CAD build for the part. Positions are in the model's coordinates, mm. Face numbers are marked on the shaded views. A direction names the side the tool comes from. Round coordinates to 2 decimals unless told otherwise and drop trailing zeros. Write each loop counter-clockwise with the first axis right and the second up, starting at its lowest first coordinate (ties: lowest second). Pieces come first, ordered by that corner, then holes. Notation, with made-up numbers: (67.25, 20.25) - (93.25, 20.25) arc R14 cw to (93.25, 24.25) - close; hole circle Ø3 at (44.5, 61). An arc over 180 degrees is marked (long way). Put each result on its own line as item: value. Start each with the question number.
Item 1: Drill centre lines: line 1 (X direction, y = 12.35, z = -58); line 2 (Z direction, x = 66.5, y = 4.5); line 3 (Z direction, x = 46.5, y = 2.5). Where is each one in solid material? Low to high. Write a range as from..to.
Item 2: Cut at B-B (z = 3). Give the cut face in (x, y).
Item 3: Cut at C-C (z = -33). Give the cut face in (x, y), and give its area (3 significant figures).
Item 4: Mould opens along Z. For the marked faces 1, 2, 3 and 4 say: released by +Z, released by -Z, zero draft, split by the parting line, or undercut.
Item 5: Cut at A-A (y = 8). Give the cut face in (x, z).
Item 6: Cut at D-D (x = 47.5). Give the cut face in (y, z).
Item 7: 3-axis set-ups, long thin cutter, end or side, ignore diameter. For the marked faces 5, 6 and 7: which of +Z, -Z, +X, -X, +Y, -Y reach the whole face in a straight line?
Item 8: Pin check, flat tips, straight feed: pin 1 Ø5 at (y, z) = (10, -6) entering from -X; pin 2 Ø4 at (x, z) = (16.5, -25.5) entering from +Y; pin 3 Ø8.5 at (x, y) = (52.5, 6) entering from +Z. Stop position of each tip, or through.
```python
from build123d import *

# Parameters (mm, degrees)
BOSS_EXTRUDE1_DEPTH          = 30
SHELL2_T                     = 3
CUT_EXTRUDE2_REACH           = 183.177
BOSS_EXTRUDE5_DEPTH          = 25.5
SKETCH17_W                   = 8
SKETCH17_H                   = 25.58
BOSS_EXTRUDE6_DEPTH          = 5
CUT_EXTRUDE3_REACH           = 182.934
SKETCH18_R                   = 1.75
SKETCH20_W                   = 197.48203017
SKETCH20_H                   = 83.172325934
CUT_EXTRUDE4_DEPTH           = 16.5
CUT_EXTRUDE5_REACH           = 180.984
OUTLINE_OF_MOTOR_PRESS_FIT_W = 41.4
OUTLINE_OF_MOTOR_PRESS_FIT_H = 20.5
SKETCH24_W                   = 46.48
SKETCH24_H                   = 2.54
BOSS_EXTRUDE7_DEPTH          = 1
CUT_EXTRUDE6_DEPTH           = 180.263074837
CUT_EXTRUDE6_DEPTH_BACK      = 180.263074837
SKETCH26_W                   = 55
SKETCH26_H                   = 13.5
BOSS_EXTRUDE8_DEPTH          = 3
FILLET1_R                    = 25
FILLET2_R                    = 25
SKETCH28_W                   = 6
SKETCH28_H                   = 6
SKETCH28_R                   = 1.75
BOSS_EXTRUDE9_DEPTH          = 2.5
FILLET3_R                    = 1
FILLET4_R                    = 10
CUT_EXTRUDE7_REACH           = 95.975
SKETCH30_R                   = 1.3


with BuildPart() as part:
    # Sketch1 → Boss-Extrude1 (new body)
    with BuildSketch(Plane(origin=(0, 0, 0), x_dir=(1, 0, 0), z_dir=(0, 1, 0))):
        Polygon((0, 46), (9, 55), (161, 55), (170, 46), (170, 9), (161, 0), (9, 0), (0, 9), align=None)
    extrude(amount=BOSS_EXTRUDE1_DEPTH)

    # Shell2 (no face opened: a closed hollow body)
    add(offset(amount=-SHELL2_T, mode=Mode.PRIVATE), mode=Mode.SUBTRACT)

    # Sketch2 → Cut-Extrude2 (cut, up to next)
    with BuildSketch(Plane(origin=(0, 30, 0), x_dir=(1, 0, 0), z_dir=(0, 1, 0)), mode=Mode.PRIVATE) as cut_extrude2_sk1:
        Polygon((3, 44.757359313), (3, 10.242640687), (10.242640687, 3), (159.757359313, 3), (167, 10.242640687), (167, 44.757359313), (159.757359313, 52), (10.242640687, 52), align=None)
    cut_extrude2_tool1 = extrude(cut_extrude2_sk1.sketch, amount=-CUT_EXTRUDE2_REACH, mode=Mode.PRIVATE) & part.part
    add(cut_extrude2_tool1.solids().sort_by_distance((85, 30, -27.5))[0], mode=Mode.SUBTRACT)

    # Sketch16 → Boss-Extrude5 (add)
    with BuildSketch(Plane(origin=(0, 3, 0), x_dir=(1, 0, 0), z_dir=(0, 1, 0))):
        Polygon((52.69, 40.29), (18.21, 40.29), (12.21, 40.29), (12.21, 37.75), (14.75, 37.75), (18.21, 37.75), (52.69, 37.75), (56.15, 37.75), (58.69, 37.75), (58.69, 40.29), align=None)
        Polygon((18.21, 17.25), (52.69, 17.25), (56.15, 17.25), (58.69, 17.25), (58.69, 14.71), (52.69, 14.71), (18.21, 14.71), (12.21, 14.71), (12.21, 17.25), (14.75, 17.25), align=None)
    extrude(amount=BOSS_EXTRUDE5_DEPTH)

    # Sketch17 → Boss-Extrude6 (add)
    with BuildSketch(Plane(origin=(0, 28.5, 0), x_dir=(1, 0, 0), z_dir=(0, 1, 0))):
        with Locations((60.192970397, 27.5)):
            Rectangle(SKETCH17_W, SKETCH17_H)
        with Locations((10.75, 27.5)):
            Rectangle(SKETCH17_W, SKETCH17_H)
    extrude(amount=-BOSS_EXTRUDE6_DEPTH)

    # Sketch18 → Cut-Extrude3 (cut, up to next)
    with BuildSketch(Plane(origin=(0, 28.5, 0), x_dir=(1, 0, 0), z_dir=(0, 1, 0)), mode=Mode.PRIVATE) as cut_extrude3_sk1:
        with Locations(Location((59.75, 32.5, 0), (0, 0, 270))):
            Circle(SKETCH18_R)
    cut_extrude3_tool1 = extrude(cut_extrude3_sk1.sketch, amount=-CUT_EXTRUDE3_REACH, mode=Mode.PRIVATE) & part.part
    # Sketch18 → Cut-Extrude3 (cut, up to next)
    with BuildSketch(Plane(origin=(0, 28.5, 0), x_dir=(1, 0, 0), z_dir=(0, 1, 0)), mode=Mode.PRIVATE) as cut_extrude3_sk2:
        with Locations(Location((59.75, 22.5, 0), (0, 0, 270))):
            Circle(SKETCH18_R)
    cut_extrude3_tool2 = extrude(cut_extrude3_sk2.sketch, amount=-CUT_EXTRUDE3_REACH, mode=Mode.PRIVATE) & part.part
    # Sketch18 → Cut-Extrude3 (cut, up to next)
    with BuildSketch(Plane(origin=(0, 28.5, 0), x_dir=(1, 0, 0), z_dir=(0, 1, 0)), mode=Mode.PRIVATE) as cut_extrude3_sk3:
        with Locations(Location((11.15, 22.5, 0), (0, 0, 270))):
            Circle(SKETCH18_R)
    cut_extrude3_tool3 = extrude(cut_extrude3_sk3.sketch, amount=-CUT_EXTRUDE3_REACH, mode=Mode.PRIVATE) & part.part
    # Sketch18 → Cut-Extrude3 (cut, up to next)
    with BuildSketch(Plane(origin=(0, 28.5, 0), x_dir=(1, 0, 0), z_dir=(0, 1, 0)), mode=Mode.PRIVATE) as cut_extrude3_sk4:
        with Locations(Location((11.15, 32.5, 0), (0, 0, 270))):
            Circle(SKETCH18_R)
    cut_extrude3_tool4 = extrude(cut_extrude3_sk4.sketch, amount=-CUT_EXTRUDE3_REACH, mode=Mode.PRIVATE) & part.part
    add(cut_extrude3_tool1.solids().sort_by_distance((59.75, 28.5, -32.5))[0], mode=Mode.SUBTRACT)
    add(cut_extrude3_tool2.solids().sort_by_distance((59.75, 28.5, -22.5))[0], mode=Mode.SUBTRACT)
    add(cut_extrude3_tool3.solids().sort_by_distance((11.15, 28.5, -22.5))[0], mode=Mode.SUBTRACT)
    add(cut_extrude3_tool4.solids().sort_by_distance((11.15, 28.5, -32.5))[0], mode=Mode.SUBTRACT)

    # Sketch20 → Cut-Extrude4 (cut)
    with BuildSketch(Plane(origin=(0, 30, 0), x_dir=(1, 0, 0), z_dir=(0, 1, 0))):
        with Locations((90.328880179, 24.260876754)):
            Rectangle(SKETCH20_W, SKETCH20_H)
    extrude(amount=-CUT_EXTRUDE4_DEPTH, mode=Mode.SUBTRACT)

    # Outline of motor press fit → Cut-Extrude5 (cut, up to next)
    with BuildSketch(Plane(origin=(0, 3, 0), x_dir=(1, 0, 0), z_dir=(0, 1, 0)), mode=Mode.PRIVATE) as cut_extrude5_sk1:
        with Locations((35.45, 27.5)):
            Rectangle(OUTLINE_OF_MOTOR_PRESS_FIT_W, OUTLINE_OF_MOTOR_PRESS_FIT_H)
    cut_extrude5_tool1 = extrude(cut_extrude5_sk1.sketch, amount=-CUT_EXTRUDE5_REACH, mode=Mode.PRIVATE) & part.part
    add(cut_extrude5_tool1.solids().sort_by_distance((35.45, 3, -27.5))[0], mode=Mode.SUBTRACT)

    # Sketch24 → Boss-Extrude7 (add)
    with BuildSketch(Plane(origin=(0, 13.5, 0), x_dir=(1, 0, 0), z_dir=(0, 1, 0))):
        with Locations((35.45, 39.02)):
            Rectangle(SKETCH24_W, SKETCH24_H)
        with Locations((35.45, 15.98)):
            Rectangle(SKETCH24_W, SKETCH24_H)
    extrude(amount=BOSS_EXTRUDE7_DEPTH)

    # Sketch25 → Cut-Extrude6 (cut, two sides: drawn at the far end of the back side and taken through both)
    with BuildSketch(Plane.XZ.offset(-CUT_EXTRUDE6_DEPTH_BACK)):
        Polygon((70, 13.461759558), (70, -84.299003111), (188.235365379, -84.299003111), (188.235365379, 23.0423143), (70, 19.718448369), align=None)
    extrude(amount=CUT_EXTRUDE6_DEPTH + CUT_EXTRUDE6_DEPTH_BACK, mode=Mode.SUBTRACT)

    # Sketch26 → Boss-Extrude8 (add)
    with BuildSketch(Plane(origin=(70, 0, 0), x_dir=(0, 0, -1), z_dir=(1, 0, 0))):
        with Locations((27.5, 6.75)):
            Rectangle(SKETCH26_W, SKETCH26_H)
    extrude(amount=-BOSS_EXTRUDE8_DEPTH)

    # Fillet1
    fillet1_edges = [part.edges().sort_by_distance(p)[0] for p in [
        (0, 6.75, -46),
        (0, 6.75, -9),
    ]]
    fillet(fillet1_edges, radius=FILLET1_R)

    # Fillet2
    # the kernel refuses this fillet: 25 mm, written as the material it takes off along each edge
    with BuildSketch(Plane(origin=(9, -18.315393785, 0), x_dir=(-0.7071067811865396, 0, -0.7071067811865553), z_dir=(0, 1, 0))) as fillet2_piece_1:
        with BuildLine():
            CenterArc((12.497293871, -22.858045188), FILLET2_R, 113.890402407, 21.109597593)
            Line((-5.180375658, -5.180375658), (-5.533929049, -4.826822268))
            Line((-5.533929049, -4.826822268), (-0.353553391, 0.353553391))
            Line((-0.353553391, 0.353553391), (0, 0.5))
            ThreePointArc((0, 0.5), (1.186291501, 0.5), (2.170088785, 0.457160904))
            Line((2.170088785, 0.457160904), (2.372583002, 0))
        make_face()
    extrude(amount=50.13078757, mode=Mode.SUBTRACT)
    with BuildSketch(Plane(origin=(9, -18.315393785, -55), x_dir=(-0.7071067811865434, 0, 0.7071067811865516), z_dir=(0, 1, 0))) as fillet2_piece_2:
        with BuildLine():
            CenterArc((12.497293871, 22.858045188), FILLET2_R, 225, 21.109597593)
            Line((-5.180375658, 5.180375658), (-5.533929049, 4.826822268))
            Line((-5.533929049, 4.826822268), (-0.353553391, -0.353553391))
            Line((-0.353553391, -0.353553391), (0, -0.5))
            ThreePointArc((0, -0.5), (1.186291501, -0.5), (2.170088785, -0.457160904))
            Line((2.170088785, -0.457160904), (2.372583002, 0))
        make_face()
    extrude(amount=50.13078757, mode=Mode.SUBTRACT)

    # Sketch28 → Boss-Extrude9 (add)
    # profile 1 of 4: a face of its own
    with BuildSketch(Plane(origin=(0, 13.5, 0), x_dir=(1, 0, 0), z_dir=(0, 1, 0))):
        with Locations((26.326157514, 58)):
            Rectangle(SKETCH28_W, SKETCH28_H)
        with Locations(Location((26.326157514, 58, 0), (0, 0, 270))):
            Circle(SKETCH28_R, mode=Mode.SUBTRACT)
    # profile 2 of 4: a face of its own
    with BuildSketch(Plane(origin=(0, 13.5, 0), x_dir=(1, 0, 0), z_dir=(0, 1, 0))):
        with Locations((57, 58)):
            Rectangle(SKETCH28_W, SKETCH28_H)
        with Locations(Location((57, 58, 0), (0, 0, 270))):
            Circle(SKETCH28_R, mode=Mode.SUBTRACT)
    # profile 3 of 4: a face of its own
    with BuildSketch(Plane(origin=(0, 13.5, 0), x_dir=(1, 0, 0), z_dir=(0, 1, 0))):
        with Locations((57, -3)):
            Rectangle(SKETCH28_W, SKETCH28_H)
        with Locations(Location((57, -3, 0), (0, 0, 270))):
            Circle(SKETCH28_R, mode=Mode.SUBTRACT)
    # profile 4 of 4: a face of its own
    with BuildSketch(Plane(origin=(0, 13.5, 0), x_dir=(1, 0, 0), z_dir=(0, 1, 0))):
        with Locations((26.326157514, -3)):
            Rectangle(SKETCH28_W, SKETCH28_H)
        with Locations(Location((26.326157514, -3, 0), (0, 0, 270))):
            Circle(SKETCH28_R, mode=Mode.SUBTRACT)
    extrude(amount=-BOSS_EXTRUDE9_DEPTH)

    # Fillet3
    fillet3_edges = [part.edges().sort_by_distance(p)[0] for p in [
        (14.75, 0, -27.5),
        (35.45, 0, -37.75),
        (56.15, 0, -27.5),
        (35.45, 0, -17.25),
        (43.163078757, 0, -55),
        (70, 0, -27.5),
        (70, 6.75, -55),
        (70, 6.75, 0),
        (0, 0, -27.5),
        (1.903011687, 0, -45.21174675),
        (1.903011687, 0, -9.78825325),
        (43.163078757, 0, 0),
        (11.746761362, 0, -54.577004107),
        (11.746761362, 0, -0.422995893),
        (23.326157514, 12.25, 0),
        (29.326157514, 12.25, 0),
        (29.326157514, 12.25, 6),
        (23.326157514, 12.25, 6),
        (60, 12.25, 0),
        (60, 12.25, 6),
        (54, 12.25, 6),
        (54, 12.25, 0),
        (54, 12.25, -55),
        (54, 12.25, -61),
        (60, 12.25, -61),
        (60, 12.25, -55),
        (29.326157514, 12.25, -55),
        (23.326157514, 12.25, -55),
        (23.326157514, 12.25, -61),
        (29.326157514, 12.25, -61),
    ]]
    fillet(fillet3_edges, radius=FILLET3_R)

    # Fillet4
    fillet4_edges = [part.edges().sort_by_distance(p)[0] for p in [
        (10.242640687, 8.25, -52),
        (3, 8.25, -44.757359313),
        (10.242640687, 8.25, -3),
        (3, 8.25, -10.242640687),
    ]]
    fillet(fillet4_edges, radius=FILLET4_R)

    # Sketch30 → Cut-Extrude7 (cut, up to next)
    with BuildSketch(Plane(origin=(70, 0, 0), x_dir=(0, 0, -1), z_dir=(1, 0, 0)), mode=Mode.PRIVATE) as cut_extrude7_sk1:
        with Locations((5.596194078, 5.596194078)):
            Circle(SKETCH30_R)
    cut_extrude7_tool1 = extrude(cut_extrude7_sk1.sketch, amount=-CUT_EXTRUDE7_REACH, mode=Mode.PRIVATE) & part.part
    # Sketch30 → Cut-Extrude7 (cut, up to next)
    with BuildSketch(Plane(origin=(70, 0, 0), x_dir=(0, 0, -1), z_dir=(1, 0, 0)), mode=Mode.PRIVATE) as cut_extrude7_sk2:
        with Locations((49.403805922, 5.596194078)):
            Circle(SKETCH30_R)
    cut_extrude7_tool2 = extrude(cut_extrude7_sk2.sketch, amount=-CUT_EXTRUDE7_REACH, mode=Mode.PRIVATE) & part.part
    add(cut_extrude7_tool1.solids().sort_by_distance((70, 5.596194, -5.596194))[0], mode=Mode.SUBTRACT)
    add(cut_extrude7_tool2.solids().sort_by_distance((70, 5.596194, -49.403806))[0], mode=Mode.SUBTRACT)


solid = part.part
```
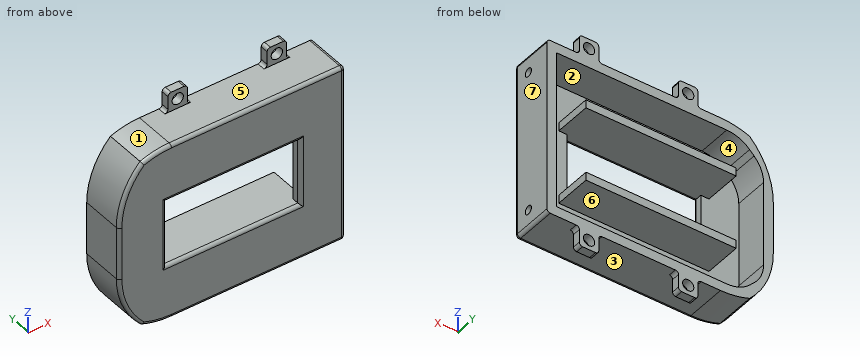
Output values:
1. line 1: 23.33..24.58, 28.08..29.33, 54..55.25, 58.75..60
1. line 2: -55..-52, -3..0
1. line 3: -55..-37.75, -17.25..0
2. outline: (23.33, 11) - (24.58, 11) - (24.58, 13.5) - (23.33, 13.5) - close; (28.08, 11) - (29.33, 11) - (29.33, 13.5) - (28.08, 13.5) - close; (54, 11) - (55.25, 11) - (55.25, 13.5) - (54, 13.5) - close; (58.75, 11) - (60, 11) - (60, 13.5) - (58.75, 13.5) - close
3. outline: (0, 1) arc R1 ccw to (1, 0) - (13.75, 0) arc R1 ccw to (14.75, 1) - (14.75, 3) - (3, 3) - (3, 13.5) - (0, 13.5) - close; (56.15, 1) arc R1 ccw to (57.15, 0) - (69, 0) arc R1 ccw to (70, 1) - (70, 13.5) - (67, 13.5) - (67, 3) - (56.15, 3) - close
3. area: 148 mm2
4. face 1: released by +Z
4. face 2: undercut
4. face 3: released by -Z
4. face 4: undercut
5. outline: (0, -35.64) arc R25 ccw to (7.32, -53.32) arc R25 ccw to (16.33, -55) - (69, -55) arc R1 ccw to (70, -54) - (70, -1) arc R1 ccw to (69, 0) - (16.33, 0) arc R25 ccw to (7.32, -1.68) arc R25 ccw to (0, -19.36) - close; (12.21, -40.29) - (58.69, -40.29) - (58.69, -37.75) - (12.21, -37.75) - close; (12.21, -17.25) - (58.69, -17.25) - (58.69, -14.71) - (12.21, -14.71) - close; hole (3, -40.62) arc R10 ccw to (5.93, -47.69) - (7.31, -49.07) arc R10 ccw to (14.38, -52) - (67, -52) - (67, -3) - (14.38, -3) arc R10 ccw to (7.31, -5.93) - (5.93, -7.31) arc R10 ccw to (3, -14.38) - close
6. outline: (0, -54) arc R1 ccw to (1, -55) - (13.5, -55) - (13.5, -52) - (3, -52) - (3, -40.29) - (14.5, -40.29) - (14.5, -37.75) - (1, -37.75) arc R1 ccw to (0, -38.75) - close; (0, -16.25) arc R1 ccw to (1, -17.25) - (14.5, -17.25) - (14.5, -14.71) - (3, -14.71) - (3, -3) - (13.5, -3) - (13.5, 0) - (1, 0) arc R1 ccw to (0, -1) - close
7. face 5: +Z, -Y
7. face 6: +Y
7. face 7: +Z, -Z, +X, +Y, -Y
8. pin 1: x = 2.48
8. pin 2: y = 3
8. pin 3: z = 0
